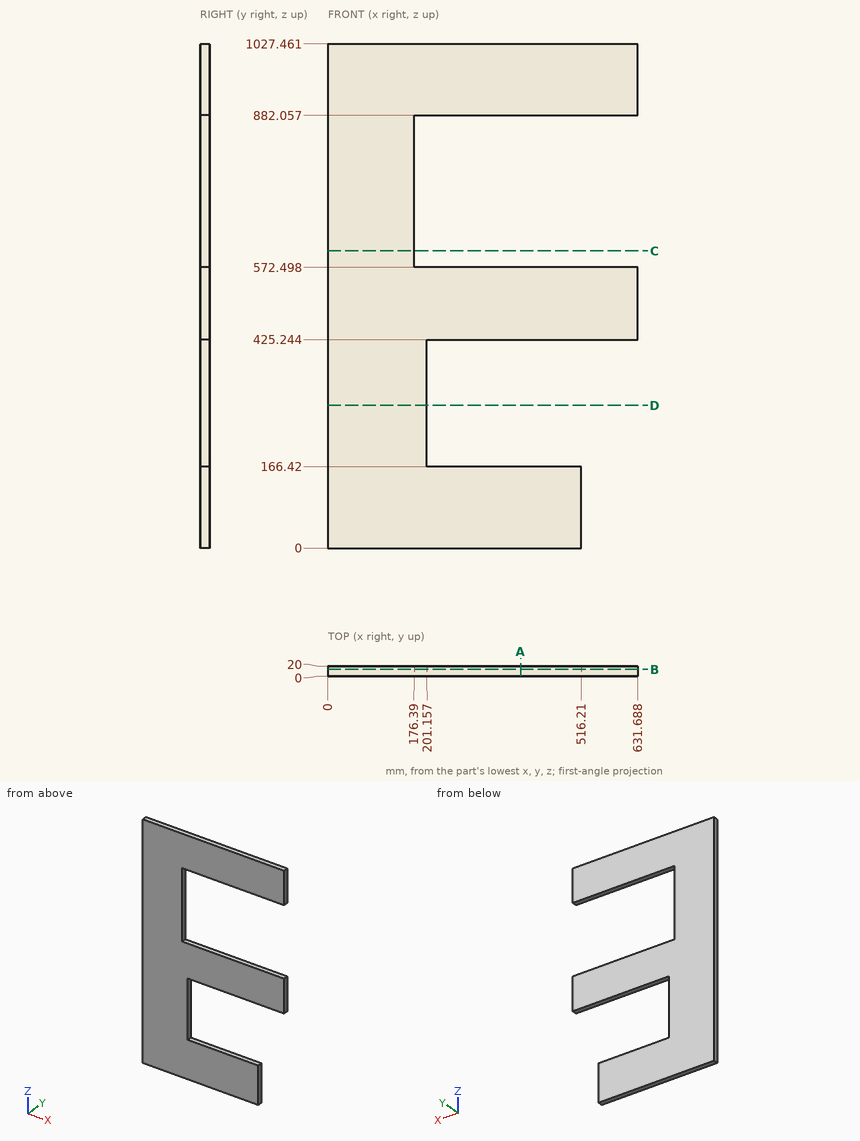
For this review, use the dimensioned drawing (mm, ordinates from the lowest corner) and the shaded views. Coordinates: 2 decimals unless noted, no trailing zeros. Write each loop counter-clockwise with the first axis right and the second up, starting at its lowest first coordinate (ties: lowest second). Pieces come first, ordered by that corner, then holes. Notation, with made-up numbers: (-26, 89.25) -> (-15, 89.25) arc R23 ccw to (-15, 97.25) -> close; hole circle Ø5 at (86.25, -13). An arc over 180 degrees is marked (long way). Put each result on its own line as item: value.
Q1. Wall thickness on L1, parallel to Z at x = 492, y = 7.5 (1 decimal); L2, parallel to Z at x = 539.5, y = 18 (1 decimal); L3, parallel to X at y = 7.5, z = 741.5: over which ranges is each line inside the solid? List them lowest first.
From the geometry:
L1: z = 0 to 166.4, 425.2 to 572.5, 882.1 to 1027.5
L2: z = 425.2 to 572.5, 882.1 to 1027.5
L3: x = 0 to 176.39
Q2. Take a section at C-C, the plane z = 606. State the section outline as (x, y) points.
From the geometry:
outline: (0, 0) -> (176.39, 0) -> (176.39, 20) -> (0, 20) -> close
Q3. Take a section at D-D, the plane z = 291. State the section outline as (x, y) points, then the cut area to 3 significant figures.
From the geometry:
outline: (0, 0) -> (201.16, 0) -> (201.16, 20) -> (0, 20) -> close
area: 4,020 mm2
Q4. Clearance check with flat-ended pins moving along their axes: pin 1 Ø10 at (y, z) = (7.5, 83.5) entering from +X; pin 2 Ø10 at (y, z) = (17, 592.5) entering from +X. State where each tip first meets the part, or that it passes through.
From the geometry:
pin 1: stops at x = 516.21
pin 2: stops at x = 176.39
Q5. Take a section at A-A, the plane x = 392.5. State the section outline as (y, z) points (1 decimal).
From the geometry:
outline: (0, 0) -> (20, 0) -> (20, 166.4) -> (0, 166.4) -> close; (0, 425.2) -> (20, 425.2) -> (20, 572.5) -> (0, 572.5) -> close; (0, 882.1) -> (20, 882.1) -> (20, 1027.5) -> (0, 1027.5) -> close
Q6. Take a section at B-B, the plane y = 13.25. State the section outline as (x, z) points (1 decimal), then the cut area to 3 significant figures.
From the geometry:
outline: (0, 0) -> (516.2, 0) -> (516.2, 166.4) -> (201.2, 166.4) -> (201.2, 425.2) -> (631.7, 425.2) -> (631.7, 572.5) -> (176.4, 572.5) -> (176.4, 882.1) -> (631.7, 882.1) -> (631.7, 1027.5) -> (0, 1027.5) -> close
area: 377,000 mm2
